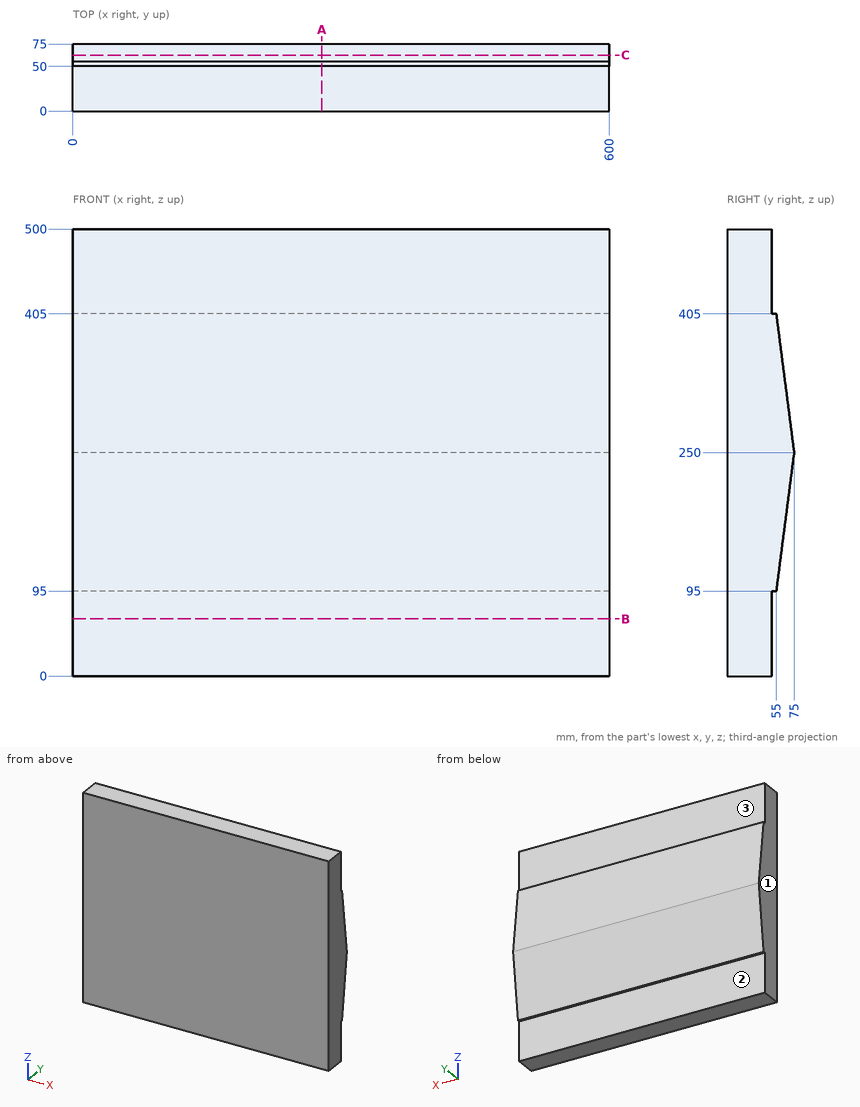
The figure shows three views and two pictorial views of one solid part (mm, origin at its lowest corner). Answer the questions. A direction names the side the tool comes from. Give positions to 0.01 mm unless a question says otherwise; leave off trailing zeros. Write each loop counter-clockwise with the first axis right and the second up, starting at its lowest first coordinate (ties: lowest second). Pieces come first, ordered by that corner, then holes. Notation, with made-up numbers: (-15, 29) -> (-5, 29) arc R12 cw to (-5, 38) -> close; hole circle Ø4 at (-29, 51.5). An arc over 180 degrees is marked (long way). Answer as a JSON object with one key per item and string values.
1) Straight lines are drawn through the part: probe 1 along Y at (x, z) = (146, 456); probe 2 along Z at (x, y) = (554, 54.5); probe 3 along Y at (x, z) = (246.5, 396.5). For each, find the intervals that lie inside material, in ascending order. Write a range as from..to.
Findings below:
{"probe 1": "y = 0..50", "probe 2": "z = 95..405", "probe 3": "y = 0..56.1"}
2) A tool of negligible diameter and unlimited length cuts with its end or side. For the marked faces 1, 2 and 3, from which of +Z, -Z, +X, -X, +Y, -Y can it reach the whole face along a straight path? Write none if from no direction.
Findings below:
{"face 1": "+Z, -Z, -X, +Y, -Y", "face 2": "-Z, +X, -X, +Y", "face 3": "+Z, +X, -X, +Y"}
3) Section C-C on y = 62.5 is taken. Write down the section's boundary in (x, z) (3 decimals).
Findings below:
{"outline": "(0, 153.125) -> (600, 153.125) -> (600, 346.875) -> (0, 346.875) -> close"}
4) Section A-A on x = 278.5 is taken. Write down the section's boundary in (y, z), then the cut area to 4 significant figures.
Findings below:
{"outline": "(0, 0) -> (50, 0) -> (50, 95) -> (55, 95) -> (75, 250) -> (55, 405) -> (50, 405) -> (50, 500) -> (0, 500) -> close", "area": "29,650 mm^2"}
5) Section B-B on z = 64 is taken. Write down the section's boundary in (x, y), then the cut area to 3 significant figures.
Findings below:
{"outline": "(0, 0) -> (600, 0) -> (600, 50) -> (0, 50) -> close", "area": "30,000 mm^2"}
6) Flat-ended cylindrical pins translate along their axes: pin 1 Ø10 at (x, z) = (381, 316) entering from +Y; pin 2 Ø12 at (x, z) = (78, 416) entering from +Y; pin 3 Ø5.5 at (x, y) = (358, 53.5) entering from +Z. Find the tip coordinate at first contact, or state that the pin passes through.
Findings below:
{"pin 1": "stops at y = 67.13", "pin 2": "stops at y = 50", "pin 3": "stops at z = 405"}
